from build123d import *

# Parameters (mm, degrees)
SKETCH2_R           = 1.6002
BOSS_EXTRUDE1_DEPTH = 4.667499936
CUT_EXTRUDE1_DEPTH  = 21.154182295
FILLET4_R           = 0.381


with BuildPart() as part:
    # Sketch2 → Boss-Extrude1 (new body)
    with BuildSketch(Plane(origin=(0, 0, 0), x_dir=(1, 0, 0), z_dir=(0, 1, 0))):
        with BuildLine():
            Line((-7.972205369, 13.335), (-7.972205369, 11.8745))
            Line((-7.972205369, 11.8745), (-12.55435155, 9.681252094))
            ThreePointArc((-12.55435155, 9.681252094), (-14.373005369, 6.7945), (-12.55435155, 3.907747906))
            Line((-12.55435155, 3.907747906), (-7.972205369, 1.7145))
            Line((-7.972205369, 1.7145), (-7.972205369, 0))
            Line((-7.972205369, 0), (7.972205369, 0))
            Line((7.972205369, 0), (7.972205369, 1.7145))
            Line((7.972205369, 1.7145), (12.55435155, 3.907747906))
            ThreePointArc((12.55435155, 3.907747906), (14.373005369, 6.7945), (12.55435155, 9.681252094))
            Line((12.55435155, 9.681252094), (7.972205369, 11.8745))
            Line((7.972205369, 11.8745), (7.972205369, 13.335))
            Line((7.972205369, 13.335), (-7.972205369, 13.335))
        make_face()
        with Locations(Location((-11.172605369, 6.7945, 0), (0, 0, 270))):
            Circle(SKETCH2_R, mode=Mode.SUBTRACT)
        with Locations(Location((11.172605369, 6.7945, 0), (0, 0, 270))):
            Circle(SKETCH2_R, mode=Mode.SUBTRACT)
    extrude(amount=BOSS_EXTRUDE1_DEPTH)

    # Sketch1 → Cut-Extrude1 (cut, through all)
    with BuildSketch(Plane.XY):
        with BuildLine():
            Line((-2.413, 4.667499936), (-5.008252596, 4.667499936))
            ThreePointArc((-5.008252596, 4.667499936), (-4.93107218, 4.666327064), (-4.853963042, 4.662809529))
            ThreePointArc((-4.853963042, 4.662809529), (-4.208266886, 4.53823071), (-3.616192862, 4.25206335))
            add(Edge.make_bspline(
                [(-3.616192862, 4.25206335), (-3.387788659, 4.102407993), (-2.866953164, 3.782649369), (-2.327154274, 3.498343868), (-2.022863606, 3.35198033)],
                knots=[0.154249258, 0.154249258, 0.154249258, 0.154249258, 0.327774555, 0.542511986, 0.542511986, 0.542511986, 0.542511986], degree=3))
            ThreePointArc((-2.022863606, 3.35198033), (-2.313410781, 3.981424459), (-2.413, 4.667499936))
        make_face()
        with BuildLine():
            Line((0, 4.667499936), (-2.413, 4.667499936))
            ThreePointArc((-2.413, 4.667499936), (-2.313410781, 3.981424459), (-2.022863606, 3.35198033))
            Line((-2.022863606, 3.35198033), (0, 3.35198033))
            Line((0, 3.35198033), (0, 4.667499936))
        make_face()
        with BuildLine():
            Line((2.413, 4.667499936), (0, 4.667499936))
            Line((0, 4.667499936), (0, 3.35198033))
            Line((0, 3.35198033), (2.022863606, 3.35198033))
            ThreePointArc((2.022863606, 3.35198033), (2.313410781, 3.981424459), (2.413, 4.667499936))
        make_face()
        with BuildLine():
            Line((0, 3.35198033), (-2.022863606, 3.35198033))
            add(Edge.make_bspline(
                [(-2.022863606, 3.35198033), (-1.011431803, 3.228904982), (0, 3.228904982)],
                knots=[0, 0, 0, 0.5, 0.5, 0.5], degree=2))
            Line((0, 3.228904982), (0, 3.35198033))
        make_face()
        with BuildLine():
            Line((2.022863606, 3.35198033), (0, 3.35198033))
            Line((0, 3.35198033), (0, 3.228904982))
            add(Edge.make_bspline(
                [(0, 3.228904982), (1.011431803, 3.228904982), (2.022863606, 3.35198033)],
                knots=[0.5, 0.5, 0.5, 1, 1, 1], degree=2))
        make_face()
        with BuildLine():
            Line((5.008252596, 4.667499936), (2.413, 4.667499936))
            ThreePointArc((2.413, 4.667499936), (2.313410781, 3.981424459), (2.022863606, 3.35198033))
            add(Edge.make_bspline(
                [(3.616192862, 4.25206335), (3.387788659, 4.102407993), (2.866953164, 3.782649369), (2.327154274, 3.498343868), (2.022863606, 3.35198033)],
                knots=[0.154249258, 0.154249258, 0.154249258, 0.154249258, 0.327774555, 0.542511986, 0.542511986, 0.542511986, 0.542511986], degree=3))
            ThreePointArc((3.616192862, 4.25206335), (4.208266886, 4.53823071), (4.853963042, 4.662809529))
            ThreePointArc((4.853963042, 4.662809529), (4.93107218, 4.666327064), (5.008252596, 4.667499936))
        make_face()
    extrude(amount=-CUT_EXTRUDE1_DEPTH, mode=Mode.SUBTRACT)

    # Fillet4
    fillet4_edges = [part.edges().sort_by_distance(p)[0] for p in [
        (0, 0, 0),
        (-6.490228982, 4.667499936, 0),
        (7.972205369, 2.333749968, 0),
        (-7.972205369, 2.333749968, 0),
        (6.490228982, 4.667499936, 0),
        (4.28188873, 4.561425887, 0),
        (2.834354543, 3.775775499, 0),
        (-4.28188873, 4.561425887, 0),
        (-2.834354543, 3.775775499, 0),
        (1.013295224, 3.259787298, 0),
    ]]
    fillet(fillet4_edges, radius=FILLET4_R)


solid = part.part
For this review, take the finished solid that the model builds, in its own axes (mm). A direction names the side the tool comes from. Coordinates: 2 decimals unless noted, no trailing zeros. Loops run counter-clockwise (first coordinate to the right, second up) from the corner with the lowest first, then second, coordinate; pieces in that order, holes last. Notation, with made-up numbers: (-10, -32) - (44, -32) arc R24 cw to (44, 5) - close; hole circle Ø6 at (61.25, 87.25). An arc over 180 degrees is marked (long way). Return JSON: item names as keys, results as strings.
Item 1: Take a section at C-C (z = -5.5). State how many separate pieces and enclosed holes the cut face has, then the cut area to 3 significant figures.
Determined:
{"separate pieces": "3", "enclosed holes": "0", "area": "105 mm2"}
Item 2: Mouldability with a two-part tool opening along X and no side actions: class faces 1 (the flat face through (-7.972, 2, -13)), 2 (the cylindrical face through (10.6, 2.3, -5.3)), 3 (the cylindrical face through (-11.79, 2.3, -5.32)), 4 (the flat face through (0, 0, -7)) as pulls with the +X half, pulls with the -X half, needs draft (parallel to the pull), parting line crosses it, or undercut.
Determined:
{"face 1": "pulls with the -X half", "face 2": "undercut", "face 3": "undercut", "face 4": "needs draft"}
Item 3: For faces 5 (the cylindrical face through (-14.373, 2.301, -6.845)), 6 (the flat face through (7.972, 2, -1)), 7 (the flat face through (-7.972, 2, -1)), 8 (the flat face through (9, 4.667, -7)), 9 (the flat face through (7.972, 2, -13)), list the 3-axis set-ups (+Z, -Z, +X, -X, +Y, -Y) from which the entire face can be reached by the end or side of a thin tool; tool diameter is ignored.
Determined:
{"face 5": "-X, +Y, -Y", "face 6": "+Z, +X, +Y, -Y", "face 7": "+Z, -X, +Y, -Y", "face 8": "+Z, -Z, +X, -X, +Y", "face 9": "-Z, +X, +Y, -Y"}
Item 4: Take a section at A-A (x = 10). Give the boundary of the cut face in (y, z).
Determined:
{"outline": "(0, -10.9) - (4.67, -10.9) - (4.67, -7.88) - (0, -7.88) - close; (0, -5.71) - (4.67, -5.71) - (4.67, -2.69) - (0, -2.69) - close"}
Item 5: Take a section at B-B (y = 1.7). Give the boundary of the cut face in (x, z) (1 decimal).
Determined:
{"outline": "(-12.6, -9.7) - (-8, -11.9) - (-8, -13.3) - (8, -13.3) - (8, -11.9) - (12.6, -9.7) arc R3.2 ccw to (12.6, -3.9) - (8, -1.7) - (8, -0.4) arc R0.4 ccw to (7.6, 0) - (-7.6, 0) arc R0.4 ccw to (-8, -0.4) - (-8, -1.7) - (-12.6, -3.9) arc R3.2 ccw to start; hole circle Ø3.2 at (-11.2, -6.8); hole circle Ø3.2 at (11.2, -6.8)"}
Item 6: Insertion check: pin 1 (0.7 mm diameter, centred on y = 2.5, z = -1, fed in from +X); pin 2 (1.6 mm diameter, centred on y = 1, z = -12.5, fed in from -X); pin 3 (6 mm diameter, centred on x = 0.5, z = -10.5, fed in from +Y). Each pin has a flat end and moves straight along its axis. Give the tip position at first contact, or say it passes through.
Determined:
{"pin 1": "stops at x = 7.97", "pin 2": "stops at x = -8.34", "pin 3": "stops at y = 4.18"}
Item 7: For line 1 (X direction, y = 4.15, z = -8); line 2 (X direction, y = 0.3, z = -5.5); line 3 (X direction, y = 3.85, z = -6.75), list the stretches that pass through material, from the lowest coordinate up.
Determined:
{"line 1": "x = -14.14 to -12.22, -10.12 to -3.46, 3.46 to 10.12, 12.22 to 14.14", "line 2": "x = -14.1 to -12.11, -10.23 to 10.23, 12.11 to 14.1", "line 3": "x = -14.37 to -12.77, -9.57 to -2.96, 2.96 to 9.57, 12.77 to 14.37"}
